from build123d import *

# Parameters (mm, degrees)
BOSS_EXTRUDE1_DEPTH      = 50.8
BOSS_EXTRUDE1_DEPTH_BACK = 50.8
SKETCH3_R                = 1.7526
CUT_EXTRUDE1_DEPTH       = 96


with BuildPart() as part:
    # Sketch1 → Boss-Extrude1 (new, two sides: drawn at the far end of the back side and taken through both)
    with BuildSketch(Plane.XY.offset(-BOSS_EXTRUDE1_DEPTH_BACK)):
        with BuildLine():
            ThreePointArc((36.411308369, -25.495472596), (0, -44.45), (-36.411308369, -25.495472596))
            Line((-36.411308369, -25.495472596), (-39.012116109, -27.316577781))
            ThreePointArc((-39.012116109, -27.316577781), (0, -47.625), (39.012116109, -27.316577781))
            Line((39.012116109, -27.316577781), (36.411308369, -25.495472596))
        make_face()
    extrude(amount=BOSS_EXTRUDE1_DEPTH + BOSS_EXTRUDE1_DEPTH_BACK)

    # Sketch3 → Cut-Extrude1 (cut)
    with BuildSketch(Plane(origin=(0, 0, 0), x_dir=(1, 0, 0), z_dir=(0, 1, 0))):
        with Locations(Location((0, 41.275, 0), (0, 0, 270))):
            Circle(SKETCH3_R)
        with Locations(Location((0, 28.636263, 0), (0, 0, 270))):
            Circle(SKETCH3_R)
        with Locations(Location((0, -28.636263, 0), (0, 0, 270))):
            Circle(SKETCH3_R)
        with Locations(Location((0, -41.275, 0), (0, 0, 270))):
            Circle(SKETCH3_R)
    extrude(amount=-CUT_EXTRUDE1_DEPTH, mode=Mode.SUBTRACT)


solid = part.part
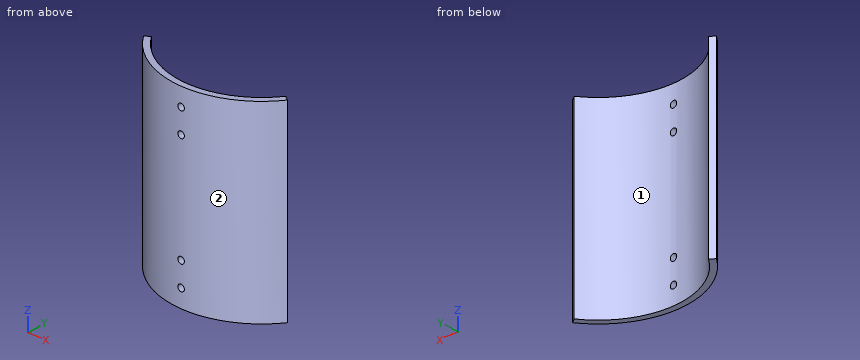
Read the model definition and answer for the solid it produces. Units are mm, in the model's axes. Face numbers are marked on the shaded views. Coordinates: 2 decimals unless noted, no trailing zeros. Write each loop counter-clockwise with the first axis right and the second up, starting at its lowest first coordinate (ties: lowest second). Pieces come first, ordered by that corner, then holes. Notation, with made-up numbers: (10, 25.25) - (59, 25.25) arc R11 cw to (59, 38.25) - close; hole circle Ø4 at (42, -19). An arc over 180 degrees is marked (long way). One line per question, with ' | ' between items.
Q1. Each of these flat-tipped pins is pushed along its axis until it touches: P1, Ø2, axis at x = 0, z = 28.64, coming from the -Y side; P2, Ø12, axis at y = -32, z = 5.5, coming from the -X side; P3, Ø1, axis at y = -31, z = -25.5, coming from the +X side; P4, Ø1.5, axis at y = -34.5, z = -29, coming from the -X side. Where does it stop, or does it pass through?
Result set:
P1: through | P2: x = -39.01 | P3: x = 36.58 | P4: x = -33.6
Q2. Find section C-C, the plane z = 37. Write down the section's boundary in (x, y) (3 decimals).
Result set:
outline: (-39.012, -27.317) arc R47.625 ccw to (39.012, -27.317) - (36.411, -25.495) arc R44.45 cw to (-36.411, -25.495) - close
Q3. Consider L1, parallel to Z at x = 0, y = -46.9; L2, parallel to Y at x = 1, z = -34.5; L3, parallel to X at y = -38.25, z = 14. Determine where each line is inside the solid, lowest interval first. Write a range as [from, to].
Result set:
L1: [-50.8, -43.03], [-39.52, -30.39], [-26.88, 26.88], [30.39, 39.52], [43.03, 50.8] | L2: [-47.61, -44.44] | L3: [-28.37, -22.64], [22.64, 28.37]
Q4. Find section B-B, the plane y = -45.5. Write down the section's boundary in (x, z) (3 decimals).
Result set:
outline: (-14.067, -50.8) - (14.067, -50.8) - (14.067, 50.8) - (-14.067, 50.8) - close; hole circle Ø3.505 at (0, -41.275); hole circle Ø3.505 at (0, -28.636); hole circle Ø3.505 at (0, 28.636); hole circle Ø3.505 at (0, 41.275)
Q5. Find section D-D, the plane x = -8. Write down the section's boundary in (y, z), plus the area to 3 significant figures.
Result set:
outline: (-46.95, -50.8) - (-43.72, -50.8) - (-43.72, 50.8) - (-46.95, 50.8) - close | area: 328 mm^2
Q6. Find section A-A, the plane x = 0. Write down the section's boundary in (y, z) (3 decimals), plus the area to 3 significant figures.
Result set:
outline: (-47.625, -50.8) - (-44.45, -50.8) - (-44.45, -43.028) - (-47.625, -43.028) - close; (-47.625, -39.522) - (-44.45, -39.522) - (-44.45, -30.389) - (-47.625, -30.389) - close; (-47.625, -26.884) - (-44.45, -26.884) - (-44.45, 26.884) - (-47.625, 26.884) - close; (-47.625, 30.389) - (-44.45, 30.389) - (-44.45, 39.522) - (-47.625, 39.522) - close; (-47.625, 43.028) - (-44.45, 43.028) - (-44.45, 50.8) - (-47.625, 50.8) - close | area: 278 mm^2
Q7. Determine the mould class of the marked faces 1 and 2 for opening direction X: +X half, -X half, draft (parallel to the pull), parting line (faces both ways), or undercut.
Result set:
face 1: undercut | face 2: parting line
